Can you work these out from the drawing? Everything is in mm from the part's minimum corner. Give positions to 0.01 mm unless a question says otherwise; leave off trailing zeros. Loops run counter-clockwise (first coordinate to the right, second up) from the corner with the lowest first, then second, coordinate; pieces in that order, holes last. Notation, with made-up numbers: (70, 16.25) - (103, 16.25) arc R19 ccw to (103, 37.25) - close; hole circle Ø7 at (-19.75, -10). An arc over 180 degrees is marked (long way). One line per item, written item: value. Start each with the question number.
Q1. If we mould it in two halves opening along Z, with no side actions, what happens to the marked faces 1, 2, 3 and 4? For each: released by +Z, released by -Z, zero draft, split by the parting line, or undercut.
Q2. If I drill on line 1 (Z direction, x = 8, y = 2) (1 decimal); line 2 (Y direction, x = 6.5, z = 3); line 3 (Y direction, x = 14.75, z = 14.5), over which ranges is the centre line in solid material (lowest first)? Write a range as from..to.
Q3. I want a section at A-A (y = 3.5). Please give me the cut outline in (x, z) (1 decimal).
Q4. I want a section at C-C (z = 54.5). Please give me the cut outline in (x, y).
Q5. I want a section at D-D (y = 6). Please give me the cut outline in (x, z) (1 decimal), then the cut area to 3 significant figures.
Q6. I'm going to push flat-ended pins straight in: P1, Ø2.5, axis at y = 5, z = 1.5, coming from the +X side (1 decimal); P2, Ø1.9, axis at x = 28.5, y = 0.5, coming from the +Z side; P3, Ø1.4, axis at x = 2, y = 1, coming from the -Z side. Where does each tip first touch, or does it pass through?
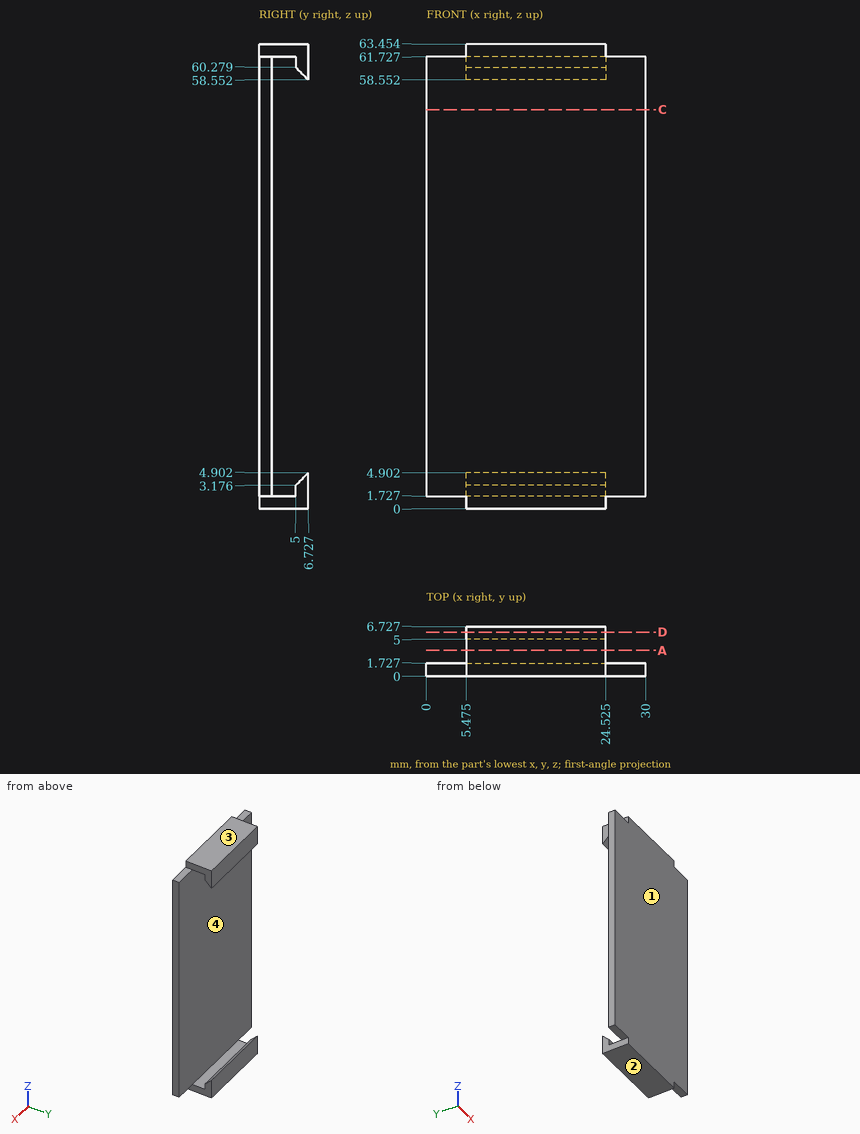
Worked answers:
1. face 1: zero draft
1. face 2: released by -Z
1. face 3: released by +Z
1. face 4: undercut
2. line 1: z = 0..1.7, 61.7..63.5
2. line 2: y = 0..1.73, 5..6.73
2. line 3: y = 0..1.73
3. outline: (5.5, 0) - (24.5, 0) - (24.5, 1.7) - (5.5, 1.7) - close; (5.5, 61.7) - (24.5, 61.7) - (24.5, 63.5) - (5.5, 63.5) - close
4. outline: (0, 0) - (30, 0) - (30, 1.73) - (0, 1.73) - close
5. outline: (5.5, 0) - (24.5, 0) - (24.5, 4.2) - (5.5, 4.2) - close; (5.5, 59.3) - (24.5, 59.3) - (24.5, 63.5) - (5.5, 63.5) - close
5. area: 159 mm²
6. P1: stops at x = 24.5
6. P2: stops at z = 61.73
6. P3: stops at z = 1.73
